Autodesk Inventor part; units mm, degrees
ref_plane "YZ Plane" through (0, 0, 0) normal (1, 0, 0) x (0, 1, 0)
ref_plane "XZ Plane" through (0, 0, 0) normal (0, 1, 0) x (-1, 0, 0)
ref_plane "XY Plane" through (0, 0, 0) normal (0, 0, 1) x (1, 0, 0)
sketch "Sketch1" plane through (0, 0, 0) normal (0, 1, 0) x (-1, 0, 0)
  circle A0 centre (0, 0) radius 16.2
  circle A1 centre (0, 0) radius 15
  dimension "d0" = 32.4
  dimension "d1" = 30
extrude "Extrusion1" add sketch "Sketch1" along normal blind 15
sketch "Sketch2" plane through (0, 0, 0) normal (1, 0, 0) x (0, 1, 0)
  line L0 (25, 0) -> (25, -8.875) construction
  line L1 (15, -16.2) -> (15, 16.2)
  line L2 (15, -16.2) -> (15, -15)
  line L3 (25, -8.875) -> (15, -15)
  line L4 (26.2, -8.875) -> (26.2, -9.34)
  line L5 (15, -16.2) -> (26.2, -9.34)
  line L6 (25, -8.875) -> (26.2, -8.875)
  line L7 (15, 0) -> (31.8321, 0)
  point P0 (0, 0)
  dimension "d7" = 1.2
revolve "Revolution1" add sketch "Sketch2" angle 360 about axis through (0, 15, 0) along (0, 1, 0)
properties part number "Top Nozzle Connector"
Can you work these out from the model? Positions are in its coordinate system, mm. A direction names the side the tool comes from. Coordinates: 2 decimals unless noted, no trailing zeros. Write each loop counter-clockwise with the first axis right and the second up, starting at its lowest first coordinate (ties: lowest second). Pieces come first, ordered by that corner, then holes. Notation, with made-up numbers: (31.25, 2) -> (70.25, 2) arc R25 cw to (70.25, 26) -> close; hole circle Ø11 at (-36.75, 79.25). An arc over 180 degrees is marked (long way). Write item = value, one per line.
(1) On a 3-axis mill with a long thin cutter (end or side, diameter ignored), from which of +Z, -Z, +X, -X, +Y, -Y can I reach the whole of each face in a straight line? I mean faces 1 (the face through (3.512, 7.395, 15.815)), 2 (the face through (14.985, 7.395, -0.66)). Say none if no direction works.
Verdict:
face_1 = +Y, -Y
face_2 = -Y
(2) Imagine slicing it at A-A (z = 0). Please give me the cut outline in (x, y) (3 decimals), and give its area (3 significant figures).
Verdict:
outline = (-16.2, 0) -> (-15, 0) -> (-15, 15) -> (-8.875, 25) -> (-8.875, 26.2) -> (-9.34, 26.2) -> (-16.2, 15) -> close; (8.875, 25) -> (15, 15) -> (15, 0) -> (16.2, 0) -> (16.2, 15) -> (9.34, 26.2) -> (8.875, 26.2) -> close
area = 62.0 mm^2
(3) For pin 1 (4 mm diameter, centred on y = 15, z = -9, fed in from -X); pin 2 (4 mm diameter, centred on y = 16.5, z = 5.5, fed in from -X); pin 3 (3 mm diameter, centred on y = 20.5, z = 6.5, fed in from +X); pin 4 (3 mm diameter, centred on x = 7.5, z = -0.5, fed in from +Y), each with a flat end and sliding along its axis, tell me the tip position at first contact or that it passes through.
Verdict:
pin_1 = -14.61
pin_2 = -15.65
pin_3 = 12.36
pin_4 = 26.2
(4) Imagine slicing it at B-B (x = 0). Please give me the cut outline in (y, z) (3 decimals), and give its area (3 significant figures).
Verdict:
outline = (0, -16.2) -> (15, -16.2) -> (26.2, -9.34) -> (26.2, -8.875) -> (25, -8.875) -> (15, -15) -> (0, -15) -> close; (0, 15) -> (15, 15) -> (25, 8.875) -> (26.2, 8.875) -> (26.2, 9.34) -> (15, 16.2) -> (0, 16.2) -> close
area = 62.0 mm^2
(5) If I drill on probe 1 along X at (y, z) = (7.5, 0); probe 2 along Z at (x, y) = (8, 21.5), over which ranges is the centre line in solid material (lowest first)?
Verdict:
probe_1 = -16.2 to -15, 15 to 16.2
probe_2 = -9.24 to -7.58, 7.58 to 9.24
(6) Imagine slicing it at C-C (y = 19.25). Please give me the cut outline in (x, z).
Verdict:
outline = circle Ø27.19 at (0, 0); hole circle Ø24.79 at (0, 0)
(7) Imagine slicing it at D-D (y = 15.5). Please give me the cut outline in (x, z).
Verdict:
outline = circle Ø31.79 at (0, 0); hole circle Ø29.39 at (0, 0)
(8) Thinking about a two-plate mould opening in X: for faces 3 (the face through (-11, 0, -11)), 4 (the face through (2.93, 25.5, -9.32)), 5 (the face through (8.664, 25.608, 1.924)), which applies, +X half, -X half, draft (parallel to the pull), parting line (faces both ways), or undercut?
Verdict:
face_3 = draft
face_4 = parting line
face_5 = undercut
